Can you work these out from the drawing? Everything is in mm from the part's minimum corner. Round coordinates to 2 decimals unless told otherwise and drop trailing zeros. Loops run counter-clockwise (first coordinate to the right, second up) from the corner with the lowest first, then second, coordinate; pieces in that order, holes last. Notation, with made-up numbers: M 30.25,42.25 L 67.25,42.25 A26 ccw 67.25,69.25 Z; hole C 58.5,28.25 d5. An arc over 180 degrees is marked long. Use a Markdown table: item, result.
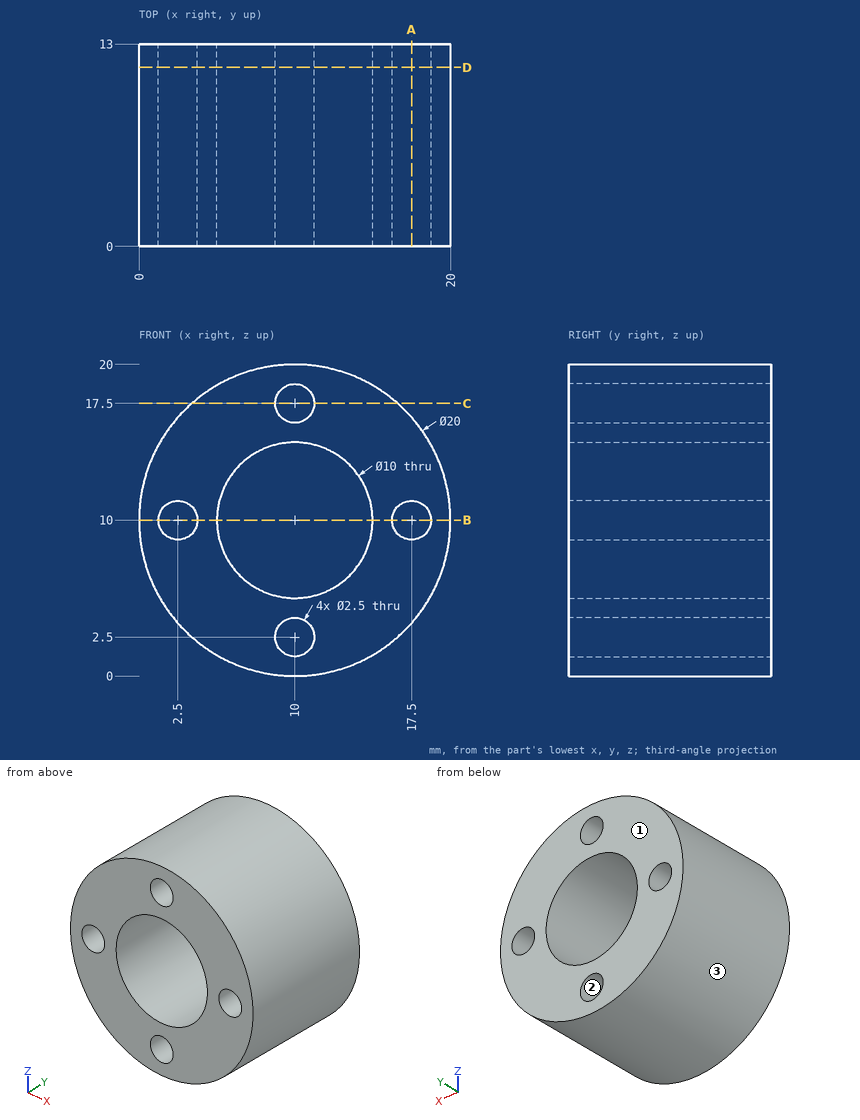
1. We'd pull the mould along Z, two halves only. Please class the marked faces 1, 2 and 3: +Z half, -Z half, draft (parallel to the pull), parting line (faces both ways), or undercut.
Answer sheet:
| item | result |
|---|---|
| face 1 | draft |
| face 2 | undercut |
| face 3 | parting line |
2. Imagine slicing it at B-B, the plane z = 10. Write out the boundary of the cut face in (x, y), then the cut area to 3 significant figures.
Answer sheet:
| item | result |
|---|---|
| outline | M 0,0 L 1.25,0 L 1.25,13 L 0,13 Z; M 3.75,0 L 5,0 L 5,13 L 3.75,13 Z; M 15,0 L 16.25,0 L 16.25,13 L 15,13 Z; M 18.75,0 L 20,0 L 20,13 L 18.75,13 Z |
| area | 65.0 mm2 |
3. Imagine slicing it at C-C, the plane z = 17.5. Write out the boundary of the cut face in (x, y), then the cut area to 3 significant figures.
Answer sheet:
| item | result |
|---|---|
| outline | M 3.39,0 L 8.75,0 L 8.75,13 L 3.39,13 Z; M 11.25,0 L 16.61,0 L 16.61,13 L 11.25,13 Z |
| area | 139 mm2 |
4. Imagine slicing it at D-D, the plane y = 11.5. Write out the boundary of the cut face in (x, z), then the cut area to 3 significant figures.
Answer sheet:
| item | result |
|---|---|
| outline | C 10,10 d20; hole C 2.5,10 d2.5; hole C 10,10 d10; hole C 10,2.5 d2.5; hole C 10,17.5 d2.5; hole C 17.5,10 d2.5 |
| area | 216 mm2 |
5. Imagine slicing it at A-A, the plane x = 17.5. Write out the boundary of the cut face in (y, z), then the cut area to 3 significant figures.
Answer sheet:
| item | result |
|---|---|
| outline | M 0,3.39 L 13,3.39 L 13,8.75 L 0,8.75 Z; M 0,11.25 L 13,11.25 L 13,16.61 L 0,16.61 Z |
| area | 139 mm2 |
6. For pin 1 Ø2 at (x, y) = (15.5, 8.5) entering from -Z; pin 2 Ø6 at (x, y) = (16.5, 6.5) entering from -Z; pin 3 Ø5 at (x, y) = (13.5, 8) entering from -Z, each with a flat end and sliding along its axis, tell me the tip position at first contact or that it passes through.
Answer sheet:
| item | result |
|---|---|
| pin 1 | z = 1.07 |
| pin 2 | z = 0.63 |
| pin 3 | z = 0.05 |
7. I need wall thicknesses on probe 1 along X at (y, z) = (10.5, 12.75); probe 2 along X at (y, z) = (7.25, 10.25); probe 3 along X at (y, z) = (1.25, 14.5). Which ranges of each line are inside material? Lowest first, please. Write a range as from..to.
Answer sheet:
| item | result |
|---|---|
| probe 1 | 0.39..5.82, 14.18..19.61 |
| probe 2 | 0..1.28, 3.72..5.01, 14.99..16.28, 18.72..20 |
| probe 3 | 1.07..7.82, 12.18..18.93 |
